Read the model definition and answer for the solid it produces. Units are mm, in the model's axes. A direction names the side the tool comes from. Give positions to 0.01 mm unless a question says otherwise; leave off trailing zeros. Write each loop counter-clockwise with the first axis right and the second up, starting at its lowest first coordinate (ties: lowest second). Pieces come first, ordered by that corner, then holes. Notation, with made-up numbers: (28, 14) -> (35, 14) arc R24 ccw to (35, 43) -> close; hole circle Ø1 at (61, -8.5). An arc over 180 degrees is marked (long way). Answer as CSV lines item,"result". Start each with the question number.
1. Find the intervals of material crossed by line 1 (X direction, y = 0, z = 0.25); line 2 (X direction, y = 0, z = -1.75); line 3 (Y direction, x = -17.5, z = 1), in increasing order.
2. The part is cut by section D-D, the plane y = 3. Determine the outline of the cut face in (x, z), and give its area (3 significant figures).
3. For a pull along Y with two mould halves and no side action, classify faces 3 (the flat face through (0, 0, 2.5)), 4 (the flat face through (0, 5, 1)), 5 (the cylindrical face through (16.524, 0.217, -0.576)) as pulls with the +Y half, pulls with the -Y half, needs draft (parallel to the pull), parting line crosses it, or undercut.
4. Given pin 1 (2 mm diameter, centred on x = -9.5, z = -2.5, fed in from -Y), flat-ended and moving along its own axis, determine where the tip first touches the part or whether it passes through.
5. The part is cut by section C-C, the plane x = -17.5. Determine the outline of the cut face in (y, z), and give its area (3 significant figures).
6. A tool of negligible diameter and unlimited length cuts with its end or side. For faces 1 (the flat face through (0, 0, 0)), 2 (the cylindrical face through (-18.476, 0.217, -0.576)), from which of +Z, -Z, +X, -X, +Y, -Y can it reach the whole face along a straight path? Write none if from no direction.
7. The part is cut by section A-A, the plane z = -1. Determine the outline of the cut face in (x, y), and give its area (3 significant figures).
8. The part is cut by section B-B, the plane y = 0. Determine the outline of the cut face in (x, z), and give its area (3 significant figures).
Solid Edge part; units mm, degrees
sketch "Sketch1" plane through (0, 0, 0) normal (0, 0, 1) x (1, 0, 0)
  line L0 (-23, -5) -> (23, -5)
  line L1 (23, -5) -> (23, 5)
  line L2 (23, 5) -> (-23, 5)
  line L3 (-23, 5) -> (-23, -5)
  dimension "D1" = 23
  dimension "D2" = 23
extrude "Protrusion1" add sketch "Sketch1" along normal blind 2.5
sketch "Sketch2" plane through (0, 0, 0) normal (0, 0, -1) x (1, 0, 0)
  line L0 (-23, 5) -> (-10.1, 5)
  line L1 (-10.1, 5) -> (-10.1, -5)
  line L2 (-10.1, -5) -> (-23, -5)
  line L3 (-23, -5) -> (-23, 5)
extrude "Base_inferiore" add sketch "Sketch2" along normal blind 3.74
mirror "Mirror1" about plane through (0, 0, 0) normal (1, 0, 0) of "Base_inferiore"
hole "Foro_2" at (17.5, 0, 2.5) direction (0, 0, -1) diameter 2 end up to next
mirror "Mirror2" about plane through (0, 0, 0) normal (1, 0, 0) of "Foro_2"
fillet "Rotondo_1" radius 0.1 2 edges at (-10.1, 0, 0) (10.1, 0, 0)
chamfer "Smusso_1" distance 0.25 angle 45 8 edges at (0, -5, 2.5) (23, 0, 2.5) (0, 5, 2.5) (-23, 0, 2.5) (-23, -5, -0.62) (23, -5, -0.62) (23, 5, -0.62) (-23, 5, -0.62)
properties part number "001"
Results found:
1,line 1,"x = -23 to -18.5, -16.5 to 16.5, 18.5 to 23"
1,line 2,"x = -23 to -18.5, -16.5 to -10.1, 10.1 to 16.5, 18.5 to 23"
1,line 3,"y = -5 to -1, 1 to 5"
2,outline,"(-23, -3.74) -> (-10.1, -3.74) -> (-10.1, -0.1) arc R0.1 cw to (-10, 0) -> (10, 0) arc R0.1 cw to (10.1, -0.1) -> (10.1, -3.74) -> (23, -3.74) -> (23, 2.25) -> (22.75, 2.5) -> (-22.75, 2.5) -> (-23, 2.25) -> close"
2,area,"211 mm²"
3,face 3,"needs draft"
3,face 4,"pulls with the +Y half"
3,face 5,"undercut"
4,pin 1,"stops at y = -5"
5,outline,"(-5, -3.74) -> (-1, -3.74) -> (-1, 2.5) -> (-4.75, 2.5) -> (-5, 2.25) -> close; (1, -3.74) -> (5, -3.74) -> (5, 2.25) -> (4.75, 2.5) -> (1, 2.5) -> close"
5,area,"49.9 mm²"
6,face 1,"-Z, +Y, -Y"
6,face 2,"+Z, -Z"
7,outline,"(-23, -4.75) -> (-22.75, -5) -> (-10.1, -5) -> (-10.1, 5) -> (-22.75, 5) -> (-23, 4.75) -> close; (10.1, -5) -> (22.75, -5) -> (23, -4.75) -> (23, 4.75) -> (22.75, 5) -> (10.1, 5) -> close; hole circle Ø2 at (-17.5, 0); hole circle Ø2 at (17.5, 0)"
7,area,"252 mm²"
8,outline,"(-23, -3.74) -> (-18.5, -3.74) -> (-18.5, 2.5) -> (-22.75, 2.5) -> (-23, 2.25) -> close; (-16.5, -3.74) -> (-10.1, -3.74) -> (-10.1, -0.1) arc R0.1 cw to (-10, 0) -> (10, 0) arc R0.1 cw to (10.1, -0.1) -> (10.1, -3.74) -> (16.5, -3.74) -> (16.5, 2.5) -> (-16.5, 2.5) -> close; (18.5, -3.74) -> (23, -3.74) -> (23, 2.25) -> (22.75, 2.5) -> (18.5, 2.5) -> close"
8,area,"186 mm²"
